Geometry: see drawing. Coordinates: mm, zero at the bounding-box minimum. Give positions to 0.01 mm unless a question says otherwise; leave off trailing zeros. Write each loop counter-clockwise with the first axis right and the second up, starting at its lowest first coordinate (ties: lowest second). Pieces come first, ordered by that corner, then holes. Notation, with made-up numbers: M -31,59.25 L -21,59.25 A22 cw -21,79.25 Z; hole C -33.75,9.5 d5. An arc over 180 degrees is marked long. Use a Markdown table: item, result. Add a question column.
(1) Cut plane C-C (z = 59). Output: boundary loops of the cut face in (x, y).
(2) Cut plane B-B (y = 1.75). Output: boundary loops of the cut face in (x, z).
(3) Cut plane A-A (z = 52). Output: boundary loops of the cut face in (x, y).
(4) Material intervals for L1, parallel to X at y = 2.05, z = 59; L2, parallel to Z at x = 27, y = 2.65; L3, parallel to X at y = 0.8, z = 19, sorted ascending.
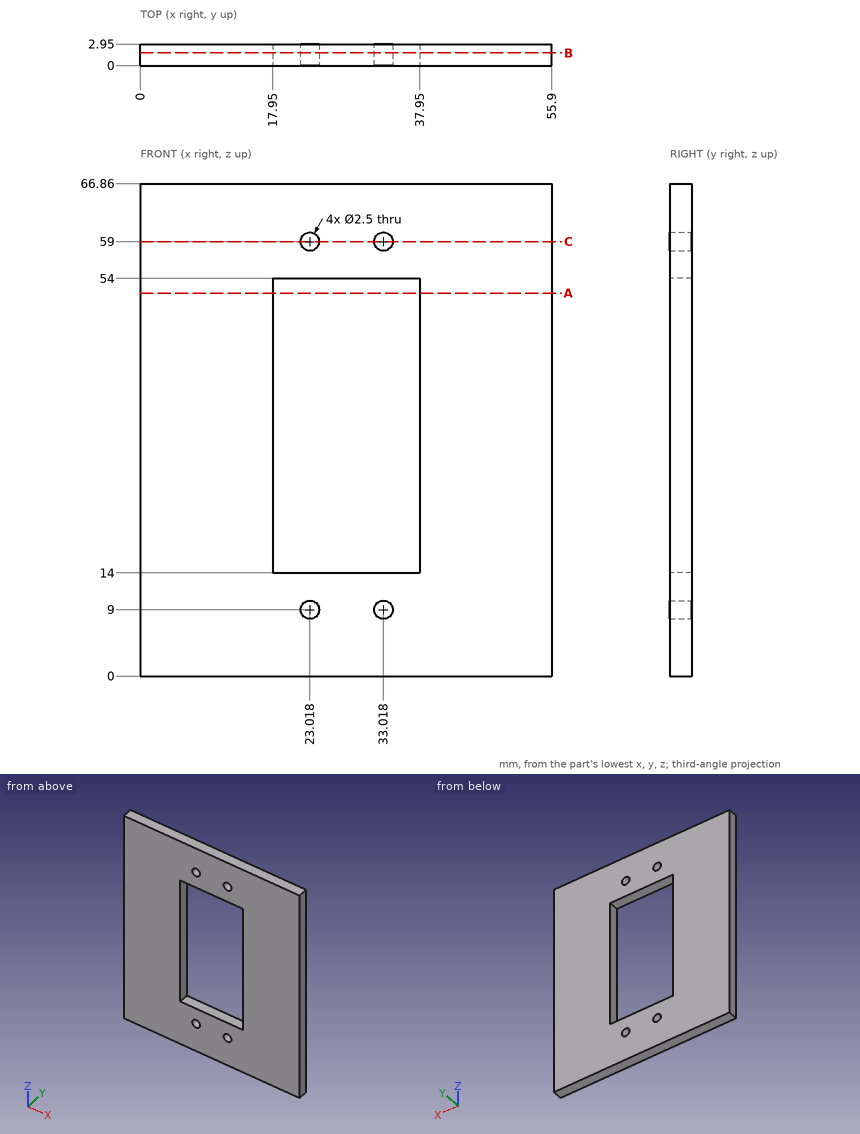
Answer list:
| question | item | result |
|---|---|---|
| 1 | outline | M 0,0 L 21.77,0 L 21.77,2.95 L 0,2.95 Z; M 24.27,0 L 31.77,0 L 31.77,2.95 L 24.27,2.95 Z; M 34.27,0 L 55.9,0 L 55.9,2.95 L 34.27,2.95 Z |
| 2 | outline | M 0,0 L 55.9,0 L 55.9,66.86 L 0,66.86 Z; hole M 17.95,14 L 37.95,14 L 37.95,54 L 17.95,54 Z; hole C 23.02,9 d2.5; hole C 23.02,59 d2.5; hole C 33.02,9 d2.5; hole C 33.02,59 d2.5 |
| 3 | outline | M 0,0 L 17.95,0 L 17.95,2.95 L 0,2.95 Z; M 37.95,0 L 55.9,0 L 55.9,2.95 L 37.95,2.95 Z |
| 4 | L1 | 0 to 21.77, 24.27 to 31.77, 34.27 to 55.9 |
| 4 | L2 | 0 to 14, 54 to 66.86 |
| 4 | L3 | 0 to 17.95, 37.95 to 55.9 |
